Source: CAD feature listing. Evaluate the final solid. Frame: model axes, mm. A direction names the side the tool comes from. Give positions to 0.01 mm unless a question says otherwise; leave off trailing zeros. Loops run counter-clockwise (first coordinate to the right, second up) from the corner with the lowest first, then second, coordinate; pieces in that order, holes last. Notation, with made-up numbers: (-6, -40) -> (0, -40) arc R26 cw to (0, -14) -> close; hole circle Ø6 at (-12.5, 51). An arc over 180 degrees is marked (long way). Answer as a JSON object with one key per item and string values. Group by question number.
from build123d import *

# Parameters (mm, degrees)
EXTRUDE_START   = 4.80128
SKETCH_1_R      = 2
EXTRUDE_1_DEPTH = 27.013538
SKETCH_2_R      = 1
EXTRUDE_2_DEPTH = 2.6
SKETCH_4_R      = 1
EXTRUDE_3_DEPTH = 2.6
EXTRUDE_START_2 = -17.963538
SKETCH_6_R      = 3.5
EXTRUDE_5_DEPTH = 7.6


with BuildPart() as part:
    # Эскиз1 → Бобышка-Вытянуть1 (new body)
    with BuildSketch(Plane.XY.offset(EXTRUDE_START)):
        Circle(SKETCH_1_R)
    extrude(amount=EXTRUDE_1_DEPTH)

    # Эскиз2 → Бобышка-Вытянуть2 (add)
    with BuildSketch(Plane.XY.offset(31.814817835)):
        Circle(SKETCH_2_R)
    extrude(amount=EXTRUDE_2_DEPTH)

    # Эскиз4 → Бобышка-Вытянуть3 (add)
    with BuildSketch(Plane(origin=(0, 0, 4.801280123), x_dir=(-1, 0, 0), z_dir=(0, 0, -1))):
        Circle(SKETCH_4_R)
    extrude(amount=EXTRUDE_3_DEPTH)

    # Эскиз6 → Бобышка-Вытянуть5 (add)
    with BuildSketch(Plane(origin=(0, 0, 4.801280123), x_dir=(-1, 0, 0), z_dir=(0, 0, -1)).offset(EXTRUDE_START_2)):
        Circle(SKETCH_6_R)
    extrude(amount=EXTRUDE_5_DEPTH)


solid = part.part
(1) Section query A-A on x = 0. Return the cut outline in (y, z), plus the area to 3 significant figures.
(2) Section query B-B on y = 0.5. Return the cut outline in (x, z), plus the area to 3 significant figures.
(3) Section query C-C on z = 25. Return the cut outline in (x, y).
(4) First-contact query: pin 1 (3 mm diameter, centred on x = -0.5, y = 2.5, fed in from -Z); pin 2 (3 mm diameter, centred on x = -2.5, z = 24, fed in from -Y); pin 3 (2 mm diameter, centred on x = 1, y = -1, fed in from -Z). Flat tips, straight axial feed; report the tip coordinate or a pass-through.
(5) Material intervals for line 1 (Z direction, x = -1.5, y = -0.5); line 2 (Z direction, x = -1.75, y = 1.5); line 3 (X direction, y = 0, z = 30), sorted ascending. Write a range as from..to.
(6) Section query D-D on z = 21.5. Return the cut outline in (x, y), plus the area to 3 significant figures.
(7) Access query for faces 1 (the face through (-2, -2, 22.765)), 2 (the face through (-3.233, -1.341, 19.018)), 3 (the face through (1, -1, 4.801)). Directions: +Z, -Z, +X, -X, +Y, -Y. A direction counts if a zero-diameter tool reaches every point of the face in a straight line with its end or side. Return the directions, or none.
Result:
{
 "1": {"outline": "(-3.5, 15.16) -> (-2, 15.16) -> (-2, 4.8) -> (-1, 4.8) -> (-1, 2.2) -> (1, 2.2) -> (1, 4.8) -> (2, 4.8) -> (2, 15.16) -> (3.5, 15.16) -> (3.5, 22.76) -> (2, 22.76) -> (2, 31.81) -> (1, 31.81) -> (1, 34.41) -> (-1, 34.41) -> (-1, 31.81) -> (-2, 31.81) -> (-2, 22.76) -> (-3.5, 22.76) -> close", "area": "141 mm²"},
 "2": {"outline": "(-3.46, 15.16) -> (-1.94, 15.16) -> (-1.94, 4.8) -> (-0.87, 4.8) -> (-0.87, 2.2) -> (0.87, 2.2) -> (0.87, 4.8) -> (1.94, 4.8) -> (1.94, 15.16) -> (3.46, 15.16) -> (3.46, 22.76) -> (1.94, 22.76) -> (1.94, 31.81) -> (0.87, 31.81) -> (0.87, 34.41) -> (-0.87, 34.41) -> (-0.87, 31.81) -> (-1.94, 31.81) -> (-1.94, 22.76) -> (-3.46, 22.76) -> close", "area": "137 mm²"},
 "3": {"outline": "circle Ø4 at (0, 0)"},
 "4": {"pin 1": "z = 4.8", "pin 2": "y = -3.09", "pin 3": "z = 2.2"},
 "5": {"line 1": "4.8..31.81", "line 2": "15.16..22.76", "line 3": "-2..2"},
 "6": {"outline": "circle Ø7 at (0, 0)", "area": "38.5 mm²"},
 "7": {"face 1": "+Z", "face 2": "+Z, -Z", "face 3": "-Z"}
}
